Geometry check sheet. Reference: drawing and pictorial views, mm from the part's lowest x, y, z. A direction names the side the tool comes from. Round coordinates to 2 decimals unless told otherwise and drop trailing zeros. Order: outer loops, then holes, each group sorted by start corner. A loop starts at its lowest first (then second) coordinate and runs counter-clockwise, first axis right, second up.
(1) Depth check by flat-ended pin: pin 1 (3 mm diameter, centred on x = 4, y = 4, fed in from +Z). Enter the tip coordinate at first touch or a pass-through.
(2) Mould release check, pull along Y, two halves, no side actions. Record for the marked faces 1, 2, 3 and 4: released by +Y, released by -Y, zero draft, split by the parting line, or undercut.
(3) Sectioned sample at C-C, the plane y = 6. Enter the section's corners in (x, z).
(4) Sectioned sample at A-A, the plane x = 3.8. Enter the section's corners in (y, z).
(5) Tool access check on the marked faces 5 and 6. Record the directions out of +Z, -Z, +X, -X, +Y, -Y that give a thin tool (end or side, any length) a straight path to the whole face; none if there is none.
(6) Thickness scan on probe 1 along X at (y, z) = (3.8, 1.65); probe 2 along Y at (x, z) = (4.75, 7). Record the ranges inside material, lowest first.
(7) Sectioned sample at D-D, the plane x = 5.75. Enter the section's corners in (y, z).
(8) Sectioned sample at B-B, the plane z = 4.5. Enter the section's corners in (x, y).
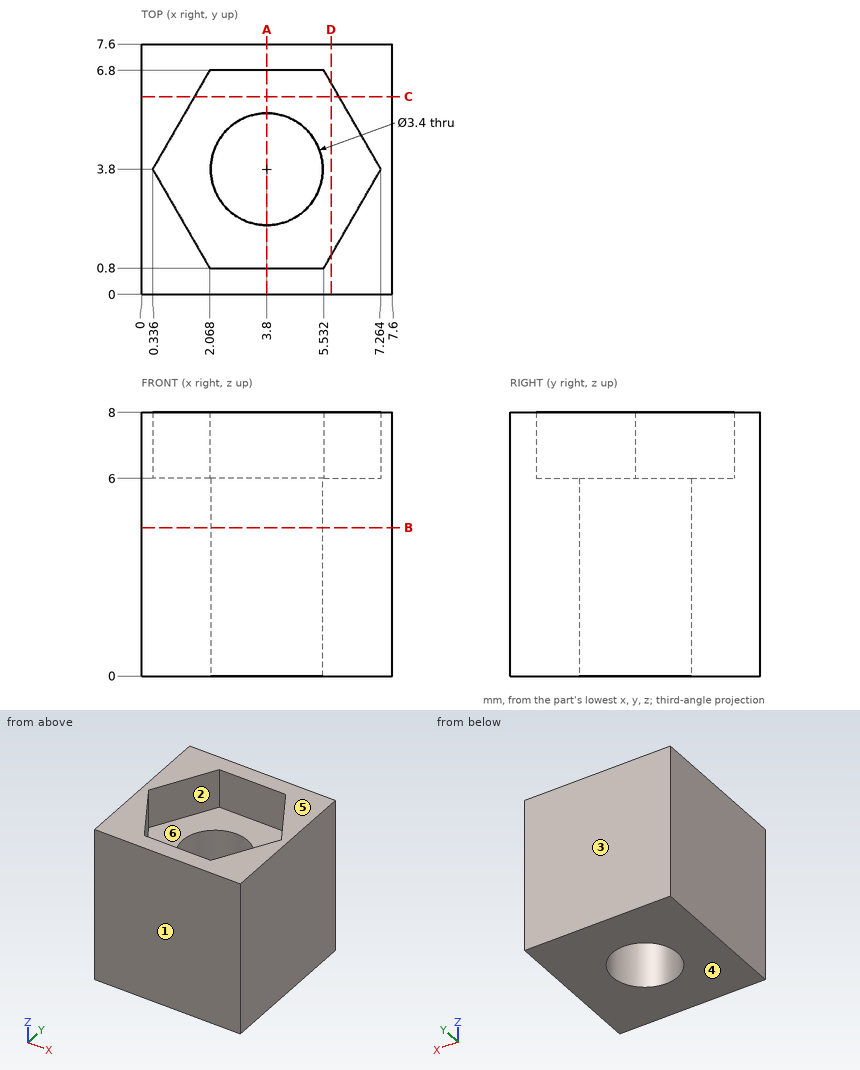
Derived:
1. pin 1: stops at z = 6
2. face 1: released by -Y
2. face 2: undercut
2. face 3: released by +Y
2. face 4: zero draft
3. outline: (0, 0) - (7.6, 0) - (7.6, 8) - (5.99, 8) - (5.99, 6) - (1.61, 6) - (1.61, 8) - (0, 8) - close
4. outline: (0, 0) - (2.1, 0) - (2.1, 6) - (0.8, 6) - (0.8, 8) - (0, 8) - close; (5.5, 0) - (7.6, 0) - (7.6, 8) - (6.8, 8) - (6.8, 6) - (5.5, 6) - close
5. face 5: +Z, +X, -X, +Y, -Y
5. face 6: +Z
6. probe 1: x = 0 to 2.1, 5.5 to 7.6
6. probe 2: y = 0 to 0.8, 6.8 to 7.6
7. outline: (0, 0) - (7.6, 0) - (7.6, 8) - (6.42, 8) - (6.42, 6) - (1.18, 6) - (1.18, 8) - (0, 8) - close
8. outline: (0, 0) - (7.6, 0) - (7.6, 7.6) - (0, 7.6) - close; hole circle Ø3.4 at (3.8, 3.8)
